Work out the finished part from the listing and answer in its coordinate system (mm). Face numbers are marked on the shaded views. A direction names the side the tool comes from. Coordinates: 2 decimals unless noted, no trailing zeros. Order: outer loops, then holes, each group sorted by start corner. A loop starts at its lowest first (then second) coordinate and runs counter-clockwise, first axis right, second up.
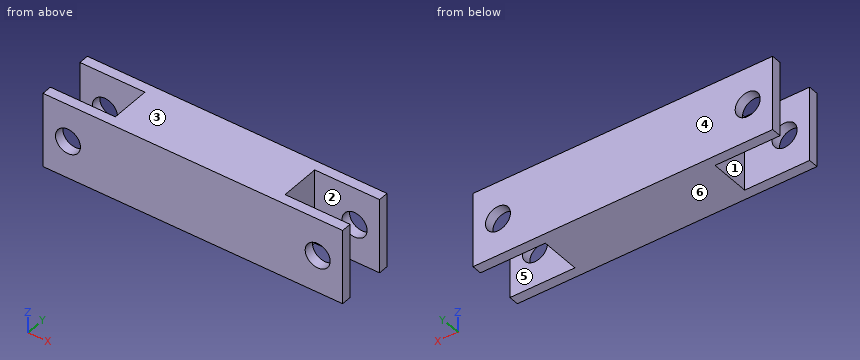
```python
from build123d import *

# Parameters (mm, degrees)
F0_W     = 300
F0_H     = 150
F0_R     = 25
F1_DEPTH = 60
F2_W     = 130
F2_H     = 150
F2_R     = 25
F3_DEPTH = 40


with BuildPart() as f1:
    # F0 (on Front) → F1 (new body, symmetric)
    with BuildSketch(Plane.XZ):
        with Locations((-150, 0)):
            Rectangle(F0_W, F0_H)
        with Locations((-250, 0)):
            Circle(F0_R, mode=Mode.SUBTRACT)
    extrude(amount=F1_DEPTH, both=True)

    # F2 (on Front) → F3 (cut, symmetric)
    with BuildSketch(Plane.XZ):
        with Locations((-235, 0)):
            Rectangle(F2_W, F2_H)
        with Locations((-250, 0)):
            Circle(F2_R, mode=Mode.SUBTRACT)
    extrude(amount=F3_DEPTH, both=True, mode=Mode.SUBTRACT)

    # F4: F1 across face


with BuildPart() as f1_1:
    add(f1.part)
    add(f1.part.mirror(Plane.YZ))


solid = f1_1.part
```
1. A flat-ended cylindrical pin translates along its axis: pin 1 (5 mm diameter, centred on y = -4, z = -54.5, fed in from -X). Find the tip coordinate at first contact, or state that the pin passes through.
2. The part is cut by section D-D (z = 65.5). Determine the outline of the cut face in (x, y), plus the area to 3 significant figures.
3. For the marked faces 1, 2 and 3, determine the directions among +Z, -Z, +X, -X, +Y, -Y from which every point of the face is accessible in a straight line to the end or side of a thin tool.
4. The mould has two halves that part along Y. Classify the marked faces 4, 5 and 6: released by +Y, released by -Y, zero draft, split by the parting line, or undercut.
5. The part is cut by section A-A (x = -250). Determine the outline of the cut face in (y, z), plus the area to 3 significant figures.
6. Consider probe 1 along Z at (x, y) = (250, -44); probe 2 along Y at (x, z) = (-189.5, -50.5); probe 3 along X at (y, z) = (0, -13.5). Determine where each line is inside the solid, lowest interval first.
7. The part is cut by section B-B (z = 0). Determine the outline of the cut face in (x, y), plus the area to 3 significant figures.
8. The part is cut by section C-C (x = 190). Determine the outline of the cut face in (y, z).
Worked out:
1. pin 1: stops at x = -170
2. outline: (-300, -60) - (300, -60) - (300, -40) - (170, -40) - (170, 40) - (300, 40) - (300, 60) - (-300, 60) - (-300, 40) - (-170, 40) - (-170, -40) - (-300, -40) - close
2. area: 51,200 mm2
3. face 1: +Z, -Z, -X
3. face 2: +Z, -Z, +X
3. face 3: +Z, +X, -X, +Y, -Y
4. face 4: released by +Y
4. face 5: undercut
4. face 6: zero draft
5. outline: (-60, -75) - (-40, -75) - (-40, -25) - (-60, -25) - close; (-60, 25) - (-40, 25) - (-40, 75) - (-60, 75) - close; (40, -75) - (60, -75) - (60, -25) - (40, -25) - close; (40, 25) - (60, 25) - (60, 75) - (40, 75) - close
5. area: 4,000 mm2
6. probe 1: z = -75 to -25, 25 to 75
6. probe 2: y = -60 to -40, 40 to 60
6. probe 3: x = -170 to 170
7. outline: (-300, -60) - (-275, -60) - (-275, -40) - (-300, -40) - close; (-300, 40) - (-275, 40) - (-275, 60) - (-300, 60) - close; (-225, -60) - (225, -60) - (225, -40) - (170, -40) - (170, 40) - (225, 40) - (225, 60) - (-225, 60) - (-225, 40) - (-170, 40) - (-170, -40) - (-225, -40) - close; (275, -60) - (300, -60) - (300, -40) - (275, -40) - close; (275, 40) - (300, 40) - (300, 60) - (275, 60) - close
7. area: 47,200 mm2
8. outline: (-60, -75) - (-40, -75) - (-40, 75) - (-60, 75) - close; (40, -75) - (60, -75) - (60, 75) - (40, 75) - close
